```python
from build123d import *

# Parameters (mm, degrees)
F0_W     = 13.335
F0_H     = 22.2504
F1_DEPTH = 12.7
F2_R     = 3.81
F3_DEPTH = 13.335


with BuildPart() as f1:
    # F0 (on Front) → F1 (new body)
    with BuildSketch(Plane.XZ):
        with Locations((6.6675, 11.1252)):
            Rectangle(F0_W, F0_H)
    extrude(amount=F1_DEPTH)

    # F2 (on Right) → F3 (join)
    with BuildSketch(Plane.YZ):
        Polygon((0, 22.2504), (0, 0), (9.491803, 0), (12.700001, 22.2504), align=None)
        with BuildLine():
            Line((0, 27.0002), (0, 22.2504))
            Line((0, 22.2504), (12.700001, 22.2504))
            Line((12.700001, 22.2504), (12.700001, 27.0002))
            ThreePointArc((12.700001, 27.0002), (6.35, 33.3502), (0, 27.0002))
        make_face()
        with Locations((6.35, 27.0002)):
            Circle(F2_R, mode=Mode.SUBTRACT)
    extrude(amount=F3_DEPTH)


solid = f1.part
```
Work out the finished part from the listing and answer in its coordinate system (mm). A direction names the side the tool comes from. Coordinates: 2 decimals unless noted, no trailing zeros. Order: outer loops, then holes, each group sorted by start corner. A loop starts at its lowest first (then second) coordinate and runs counter-clockwise, first axis right, second up. Notation, with made-up numbers: (42.5, 53) - (81.5, 53) arc R15 cw to (81.5, 64) - close; hole circle Ø5 at (-34.5, 47). An arc over 180 degrees is marked (long way). Answer as a JSON object with one key per item and string values.
1. Find section A-A on x = 4. Determine the outline of the cut face in (y, z).
Output values:
{"outline": "(-12.7, 0) - (9.49, 0) - (12.7, 22.25) - (12.7, 27) arc R6.35 ccw to (0, 27) - (0, 22.25) - (-12.7, 22.25) - close; hole circle Ø7.62 at (6.35, 27)"}
2. Each of these flat-tipped pins is pushed along its axis until it touches: P1, Ø1, axis at x = 9, y = -2, coming from the +Z side; P2, Ø5, axis at x = 9, z = 25.5, coming from the -Y side; P3, Ø2, axis at x = 1.5, z = 12, coming from the +Y side. Where does it stop, or does it pass through?
Output values:
{"P1": "stops at z = 22.25", "P2": "stops at y = 0", "P3": "stops at y = 11.37"}
3. Find section C-C on z = 29. Determine the outline of the cut face in (x, y) (3 decimals).
Output values:
{"outline": "(0, 0.323) - (13.335, 0.323) - (13.335, 3.107) - (0, 3.107) - close; (0, 9.593) - (13.335, 9.593) - (13.335, 12.377) - (0, 12.377) - close"}
4. A tool of negligible diameter and unlimited length cuts with its end or side. For faces 1 (the face through (13.335, 0, 13)), 2 (the face through (7, 0, 25)), from which of +Z, -Z, +X, -X, +Y, -Y can it reach the whole face along a straight path? Write none if from no direction.
Output values:
{"face 1": "+Z, -Z, +X, +Y, -Y", "face 2": "+Z, +X, -X, -Y"}
5. The mould has two halves that part along Z. Classify faces 3 (the face through (7, -12.7, 11)), 4 (the face through (7, -6, 22.25)), 5 (the face through (6.574, 5.854, 30.778)): +Z half, -Z half, draft (parallel to the pull), parting line (faces both ways), or undercut.
Output values:
{"face 3": "draft", "face 4": "+Z half", "face 5": "undercut"}
6. Find section D-D on y = -2.25. Determine the outline of the cut face in (x, z) (3 decimals).
Output values:
{"outline": "(0, 0) - (13.335, 0) - (13.335, 22.25) - (0, 22.25) - close"}
7. Consider line 1 (Z direction, x = 4, y = 6.35); line 2 (Z direction, x = 5, y = 8.5); line 3 (Z direction, x = 2, y = -1). Determine where each line is inside the solid, lowest interval first.
Output values:
{"line 1": "z = 0 to 23.19, 30.81 to 33.35", "line 2": "z = 0 to 23.85, 30.15 to 32.98", "line 3": "z = 0 to 22.25"}
8. Find section B-B on y = 6.35. Determine the outline of the cut face in (x, z) (3 decimals).
Output values:
{"outline": "(0, 0) - (13.335, 0) - (13.335, 23.19) - (0, 23.19) - close; (0, 30.81) - (13.335, 30.81) - (13.335, 33.35) - (0, 33.35) - close"}
